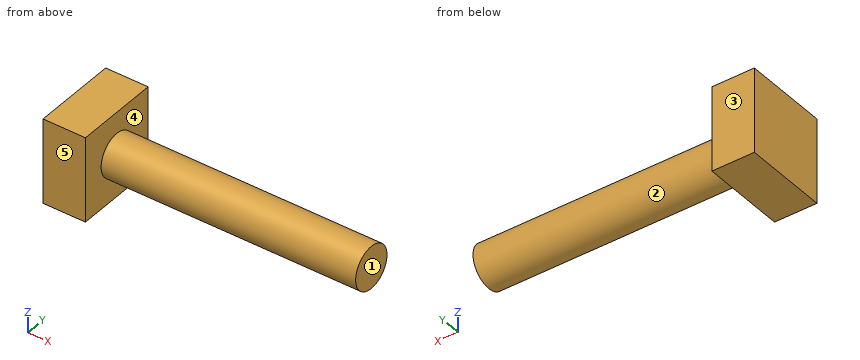
```python
from build123d import *

# Parameters (mm, degrees)
F0_W     = 25.4
F0_H     = 25.4
F1_DEPTH = 12.7
F2_R     = 6.35
F3_DEPTH = 76.2


with BuildPart() as f1:
    # F0 (on Right) → F1 (new body)
    with BuildSketch(Plane.YZ):
        Rectangle(F0_W, F0_H)
    extrude(amount=F1_DEPTH)

    # F2 (on face) → F3 (join)
    with BuildSketch(Plane.YZ.offset(12.7)):
        Circle(F2_R)
    extrude(amount=F3_DEPTH)


solid = f1.part
```
Can you work these out from the model? Positions are in its coordinate system, mm. Face numbers are marked on the shaded views. A direction names the side the tool comes from. Give positions to 0.01 mm unless a question says otherwise; leave off trailing zeros. Loops run counter-clockwise (first coordinate to the right, second up) from the corner with the lowest first, then second, coordinate; pieces in that order, holes last. Notation, with made-up numbers: M -17.5,-17 L 31.5,-17 A12 ccw 31.5,2 Z; hole C 10,33 d5. An arc over 180 degrees is marked long. One line per item, written item: value.
(1) We'd pull the mould along Y, two halves only. Please class the marked faces 3, 4 and 5: released by +Y, released by -Y, zero draft, split by the parting line, or undercut.
Returned:
face 3: released by +Y
face 4: zero draft
face 5: released by -Y
(2) Will these pins go through, and if not, where does the flat tip stop? pin 1 (1 mm diameter, centred on y = 8, z = 1.5, fed in from +X); pin 2 (2 mm diameter, centred on x = 19, y = 5.5, fed in from +Z); pin 3 (8 mm diameter, centred on x = 19.5, y = 2, fed in from -Z); pin 4 (12.5 mm diameter, centred on y = 6.5, z = -4.5, fed in from +X).
Returned:
pin 1: x = 12.7
pin 2: z = 4.48
pin 3: z = -6.35
pin 4: x = 88.9
(3) Which directions (+Z, -Z, +X, -X, +Y, -Y) give clear straight access to the entire face, cutting with the end or side of a thin tool? Please do the marked faces 1 and 2.
Returned:
face 1: +Z, -Z, +X, +Y, -Y
face 2: +X
(4) Suppose I cut it at D-D on z = 10.5. List the corners of the cut face in (x, y) for me, plus the area to 3 significant figures.
Returned:
outline: M 0,-12.7 L 12.7,-12.7 L 12.7,12.7 L 0,12.7 Z
area: 323 mm^2
(5) Suppose I cut it at C-C on x = 47. List the corners of the cut face in (y, z) for me.
Returned:
outline: C 0,0 d12.7
(6) Suppose I cut it at A-A on z = 0. List the corners of the cut face in (x, y) for me, plus the area to 3 significant figures.
Returned:
outline: M 0,-12.7 L 12.7,-12.7 L 12.7,-6.35 L 88.9,-6.35 L 88.9,6.35 L 12.7,6.35 L 12.7,12.7 L 0,12.7 Z
area: 1,290 mm^2
(7) I need wall thicknesses on line 1 (Y direction, x = 75, z = 0.25); line 2 (X direction, y = 11.5, z = -0.25); line 3 (Z direction, x = 13, y = -0.5). Which ranges of each line are inside material? Lowest first, please.
Returned:
line 1: -6.35 to 6.35
line 2: 0 to 12.7
line 3: -6.33 to 6.33
